Read the model definition and answer for the solid it produces. Units are mm, in the model's axes. Coordinates: 2 decimals unless noted, no trailing zeros. Write each loop counter-clockwise with the first axis right and the second up, starting at its lowest first coordinate (ties: lowest second). Pieces come first, ordered by that corner, then holes.
(1) Find the intervals of material crossed by probe 1 along X at (y, z) = (3.5, 0.5); probe 2 along Y at (x, z) = (-12, 0.75); probe 3 along Y at (x, z) = (-13.5, 2.5), in increasing order.
(2) The mould has two halves that part along X. Classify faces 1 (the cylindrical face through (41.986, 0.193, -0.046)), 2 (the cylindrical face through (-10.37, -25.22, 2.96)), 3 (the flat face through (24, -10.662, 0)), 4 (the cylindrical face through (-27.39, -30.16, -0.05)): +X half, -X half, draft (parallel to the pull), parting line (faces both ways), or undercut.
(3) Section A-A on z = 0.5 is taken. Write down the section's boundary in (x, y).
(4) Given pin 1 (2 mm diameter, centred on y = 7.5, z = -0.5, fed in from -X); pin 2 (2 mm diameter, centred on x = 19.5, z = -0.5, fed in from -Y); pin 3 (12 mm diameter, centred on x = 24.5, y = -16.5, fed in from +Z), each flat-ended and moving along its own axis, determine where each tip first touches the part or whether it passes through.
Autodesk Inventor part; units mm, degrees
ref_plane "YZ Plane" through (0, 0, 0) normal (1, 0, 0) x (0, 1, 0)
ref_plane "XZ Plane" through (0, 0, 0) normal (0, 1, 0) x (-1, 0, 0)
ref_plane "XY Plane" through (0, 0, 0) normal (0, 0, 1) x (1, 0, 0)
sketch "Sketch1" plane through (0, 0, 0) normal (0, 0, 1) x (1, 0, 0)
  arc A0 (-36.3497, -18.0713) -> (-15.9827, -32.4309) centre (-25.5909, -24.4351) ccw
  arc A1 (35.8842, -10.6617) -> (38.9651, 7.8249) centre (35.8842, -1.1617) ccw
  arc A2 (-1.287, 21.6247) -> (-16.0996, 16.1641) centre (-5.3408, 9.8003) ccw
  arc A3 (12.4467, -10.6617) -> (-4.4637, -18.5891) centre (12.4467, -32.6617) ccw
  line L0 (-15.9827, -32.4309) -> (-4.4637, -18.5891)
  line L1 (12.4467, -10.6617) -> (35.8842, -10.6617)
  line L2 (38.9651, 7.8249) -> (-1.287, 21.6247)
  line L3 (-16.0996, 16.1641) -> (-36.3497, -18.0713)
  dimension "d0" = 12.5
  dimension "d1" = 9.5
  dimension "d2" = 12.5
  dimension "d3" = 22
extrude "Extrusion1" add sketch "Sketch1" along normal mid plane 6.5
sketch "Sketch2" plane through (0, 0, 3.25) normal (0, 0, 1) x (1, 0, 0)
  arc A0 (-36.3497, -18.0713) -> (-15.9827, -32.4309) centre (-25.5909, -24.4351) ccw
  arc A1 (-1.287, 21.6247) -> (-16.0996, 16.1641) centre (-5.3408, 9.8003) ccw
  arc A2 (35.8842, -10.6617) -> (38.9651, 7.8249) centre (35.8842, -1.1617) ccw
  line L0 (-36.3497, -18.0713) -> (-16.0996, 16.1641)
  line L1 (-4.4637, -18.5891) -> (-15.9827, -32.4309)
  arc A3 (12.4467, -10.6617) -> (-4.4637, -18.5891) centre (12.4467, -32.6617) ccw
  line L2 (35.8842, -10.6617) -> (12.4467, -10.6617)
  line L3 (-1.287, 21.6247) -> (38.9651, 7.8249)
hole "Hole1" at (-25.5909, -24.4351, 3.25) direction (0, 0, -1) diameter 12 end through all
sketch "Sketch3" plane through (0, 0, 3.25) normal (0, 0, 1) x (1, 0, 0)
  arc A0 (-1.287, 21.6247) -> (-16.0996, 16.1641) centre (-5.3408, 9.8003) ccw
hole "Hole2" at (-5.3408, 9.8003, 3.25) direction (0, 0, -1) diameter 19 end through all
sketch "Sketch4" plane through (0, 0, 3.25) normal (0, 0, 1) x (1, 0, 0)
  arc A0 (35.8842, -10.6617) -> (38.9651, 7.8249) centre (35.8842, -1.1617) ccw
hole "Hole3" at (35.8842, -1.1617, 3.25) direction (0, 0, -1) diameter 12.5 end through all
fillet "Fillet1" radius 1 16 edges at (18.8391, 14.7248, 3.25) (45.2549, -2.7234, 3.25) (24.1654, -10.6617, 3.25) (3.1086, -12.7419, 3.25) (-10.2232, -25.51, 3.25) (-32.7937, -34.6512, 3.25) (-26.2246, -0.9536, 3.25) (-9.6644, 21.5287, 3.25) (18.8391, 14.7248, -3.25) (-9.6644, 21.5287, -3.25) (-26.2246, -0.9536, -3.25) (-32.7937, -34.6512, -3.25) (-10.2232, -25.51, -3.25) (3.1086, -12.7419, -3.25) (24.1654, -10.6617, -3.25) (45.2549, -2.7234, -3.25)
properties part number "WeldExer_base"
Response:
1. probe 1: x = -23.59 to -12.45, 1.77 to 31.72, 40.05 to 44.16
1. probe 2: y = -27.65 to 3.02, 16.58 to 20.38
1. probe 3: y = -29.4 to 4.93, 14.67 to 19.23
2. face 1: undercut
2. face 2: +X half
2. face 3: draft
2. face 4: undercut
3. outline: (-36.35, -18.07) arc R12.5 ccw to (-15.98, -32.43) - (-4.46, -18.59) arc R22 cw to (12.45, -10.66) - (35.88, -10.66) arc R9.5 ccw to (38.97, 7.82) - (-1.29, 21.62) arc R12.5 ccw to (-16.1, 16.16) - close; hole circle Ø12 at (-25.59, -24.44); hole circle Ø19 at (-5.34, 9.8); hole circle Ø12.5 at (35.88, -1.16)
4. pin 1: stops at x = -21.82
4. pin 2: stops at y = -10.66
4. pin 3: stops at z = 2.8
